```python
from build123d import *

# Parameters (mm, degrees)
SKETCH013_W  = 51
SKETCH013_H  = 5
PAD011_DEPTH = 8
SKETCH014_W  = 65
SKETCH014_H  = 30.7
SKETCH014_R  = 1.375
PAD012_DEPTH = 1.651
FILLET003_R  = 3.5
SKETCH017_W  = 10
SKETCH017_H  = 10
PAD014_DEPTH = 3.15
SKETCH018_R  = 2.975
PAD015_DEPTH = 2.65
SKETCH019_W  = 3.2
SKETCH019_H  = 3.2
PAD016_DEPTH = 2.8
SKETCH020_W  = 6
SKETCH020_H  = 6
PAD017_DEPTH = 1.8
SKETCH021_R  = 1.5
PAD018_DEPTH = 1.3
SKETCH022_W  = 26
SKETCH022_H  = 30
PAD019_DEPTH = 1.65


with BuildPart() as part:
    # Sketch013 → Pad011 (new body)
    with BuildSketch(Plane.XY):
        with Locations((32.5, -3)):
            Rectangle(SKETCH013_W, SKETCH013_H)
    extrude(amount=PAD011_DEPTH)

    # Sketch014 (on Face6 of Pad011) → Pad012 (join)
    with BuildSketch(Plane.XY.offset(8)):
        with Locations((32.5, -15.35)):
            Rectangle(SKETCH014_W, SKETCH014_H)
        with Locations((3.5, -3.5)):
            Circle(SKETCH014_R, mode=Mode.SUBTRACT)
        with Locations((61.5, -3.5)):
            Circle(SKETCH014_R, mode=Mode.SUBTRACT)
        with Locations((61.5, -26.5)):
            Circle(SKETCH014_R, mode=Mode.SUBTRACT)
        with Locations((3.5, -26.5)):
            Circle(SKETCH014_R, mode=Mode.SUBTRACT)
    extrude(amount=PAD012_DEPTH)

    # Fillet003
    fillet003_edges = [part.edges().sort_by_distance(p)[0] for p in [
        (0, 0, 8.8255),
        (0, -30.7, 8.8255),
        (65, -30.7, 8.8255),
        (65, 0, 8.8255),
    ]]
    fillet(fillet003_edges, radius=FILLET003_R)

    # Sketch017 (on Face5 of Fillet003) → Pad014 (join)
    with BuildSketch(Plane.XY.offset(9.651)):
        with Locations((8, -17.24)):
            Rectangle(SKETCH017_W, SKETCH017_H)
    extrude(amount=PAD014_DEPTH)

    # Sketch018 (on Face24 of Pad014) → Pad015 (join)
    with BuildSketch(Plane.XY.offset(12.801)):
        with Locations((8, -17.24)):
            Circle(SKETCH018_R)
    extrude(amount=PAD015_DEPTH)

    # Sketch019 (on Face26 of Pad015) → Pad016 (join)
    with BuildSketch(Plane.XY.offset(15.451)):
        with Locations((8, -17.24)):
            Rectangle(SKETCH019_W, SKETCH019_H)
    extrude(amount=PAD016_DEPTH)

    # Sketch020 (on Face5 of Pad016) → Pad017 (join)
    with BuildSketch(Plane.XY.offset(9.651)):
        with Locations((61.09, -14.95)):
            Rectangle(SKETCH020_W, SKETCH020_H)
        with Locations((53.75, -21.43)):
            Rectangle(SKETCH020_W, SKETCH020_H)
    extrude(amount=PAD017_DEPTH)

    # Sketch021 (on Face34 of Pad017) → Pad018 (join)
    with BuildSketch(Plane.XY.offset(11.451)):
        with Locations((53.75, -21.43)):
            Circle(SKETCH021_R)
        with Locations((61.09, -14.95)):
            Circle(SKETCH021_R)
    extrude(amount=PAD018_DEPTH)

    # Sketch022 (on Face5 of Pad018) → Pad019 (join)
    with BuildSketch(Plane.XY.offset(9.651)):
        with Locations((32.51, -15.7)):
            Rectangle(SKETCH022_W, SKETCH022_H)
    extrude(amount=PAD019_DEPTH)


with BuildPart() as part_1:
    # Body002 placement: moved
    add(part.part.moved(Location((0, 0, 4))))


solid = part_1.part
```
Work out the finished part from the listing and answer in its coordinate system (mm). A direction names the side the tool comes from. Give positions to 0.01 mm unless a question says otherwise; leave off trailing zeros. Loops run counter-clockwise (first coordinate to the right, second up) from the corner with the lowest first, then second, coordinate; pieces in that order, holes last. Notation, with made-up numbers: (-13, -9) -> (41, -9) arc R27 ccw to (41, 25) -> close; hole circle Ø5 at (45.5, -10). An arc over 180 degrees is marked (long way). Put each result on its own line as item: value. Start each with the question number.
Item 1: The mould has two halves that part along X. Classify faces 5 (the face through (63.95, -1, 12.84)), 6 (the face through (6.4, -17, 21)), 7 (the face through (46, -15, 13.651)), 8 (the face through (54, -21, 16.751)): released by +X, released by -X, zero draft, split by the parting line, or undercut.
Item 2: The part is cut by section B-B (y = -17.24). Give the vertices of the cut face in (x, z) (3 decimals), then the cut area to 3 significant figures.
Item 3: Find the intervals of material crossed by L1, parallel to Y at x = 3.5, z = 12.5 (3 decimals); L2, parallel to X at y = -2, z = 10.75; L3, parallel to Z at x = 44.5, y = -13, in increasing order. Write a range as [from, to].
Item 4: Each of these flat-tipped pins is pushed along its axis until it touches: P1, Ø3, axis at x = 61.5, y = -3.5, coming from the +Z side; P2, Ø1.5, axis at y = -4, z = 8, coming from the -X side; P3, Ø0.5, axis at x = 52.5, z = 15, coming from the -Y side. Where does it stop, or does it pass through?
Item 5: The part is cut by section C-C (y = -26.5). Give the vertices of the cut face in (x, z) (3 decimals), then the cut area to 3 significant figures.
Item 6: Which of the six approach directions +Z, -Z, +X, -X, +Y, -Y give full straight-line access (tool end or side, diameter ignored) to faces 1 (the face through (10.2, -14.9, 16.801)), 2 (the face through (64.09, -15, 15)), 3 (the face through (19.51, -16, 14)), 4 (the face through (8, -15.64, 21))?
Item 7: The part is cut by section D-D (x = 8). Give the vertices of the cut face in (y, z) (3 decimals).
Item 8: The part is cut by section A-A (x = 22). Give the vertices of the cut face in (y, z).
Answers below:
1. face 5: released by +X
1. face 6: released by -X
1. face 7: undercut
1. face 8: zero draft
2. outline: (0, 12) -> (65, 12) -> (65, 13.651) -> (64.09, 13.651) -> (64.09, 15.451) -> (58.09, 15.451) -> (58.09, 13.651) -> (45.51, 13.651) -> (45.51, 15.301) -> (19.51, 15.301) -> (19.51, 13.651) -> (13, 13.651) -> (13, 16.801) -> (10.975, 16.801) -> (10.975, 19.451) -> (9.6, 19.451) -> (9.6, 22.251) -> (6.4, 22.251) -> (6.4, 19.451) -> (5.025, 19.451) -> (5.025, 16.801) -> (3, 16.801) -> (3, 13.651) -> (0, 13.651) -> close
2. area: 217 mm2
3. L1: [-30.7, -27.875], [-25.125, -4.875], [-2.125, 0]
3. L2: [7, 58]
3. L3: [12, 15.3]
4. P1: z = 13.65
4. P2: x = 7
4. P3: y = -24.43
5. outline: (0, 12) -> (2.125, 12) -> (2.125, 13.651) -> (0, 13.651) -> close; (4.875, 12) -> (60.125, 12) -> (60.125, 13.651) -> (45.51, 13.651) -> (45.51, 15.301) -> (19.51, 15.301) -> (19.51, 13.651) -> (4.875, 13.651) -> close; (62.875, 12) -> (65, 12) -> (65, 13.651) -> (62.875, 13.651) -> close
5. area: 141 mm2
6. face 1: +Z
6. face 2: +Z, +X, +Y, -Y
6. face 3: +Z, +Y, -Y
6. face 4: +Z, +X, -X, +Y
7. outline: (-30.7, 12) -> (-5.5, 12) -> (-5.5, 4) -> (-0.5, 4) -> (-0.5, 12) -> (0, 12) -> (0, 13.651) -> (-12.24, 13.651) -> (-12.24, 16.801) -> (-14.265, 16.801) -> (-14.265, 19.451) -> (-15.64, 19.451) -> (-15.64, 22.251) -> (-18.84, 22.251) -> (-18.84, 19.451) -> (-20.215, 19.451) -> (-20.215, 16.801) -> (-22.24, 16.801) -> (-22.24, 13.651) -> (-30.7, 13.651) -> close
8. outline: (-30.7, 12) -> (-5.5, 12) -> (-5.5, 4) -> (-0.5, 4) -> (-0.5, 12) -> (0, 12) -> (0, 13.65) -> (-0.7, 13.65) -> (-0.7, 15.3) -> (-30.7, 15.3) -> close
